Solid Edge part; units mm, degrees
sketch "Sketch1" plane through (0, 0, 0) normal (0, 0, 1) x (1, 0, 0)
  circle A0 centre (0, 0) radius 32
extrude "Protrusion1" add sketch "Sketch1" against normal blind 8
sketch "Sketch2" plane through (0, 0, 0) normal (0, 0, 1) x (1, 0, 0)
  circle A0 centre (0, 0) radius 10
extrude "nucleo" add sketch "Sketch2" along normal blind 3
sketch "Sketch3" plane through (0, 0, -8) normal (0, 0, -1) x (-1, 0, 0)
  line L0 (-9.0257, 1.3213) -> (-30.1049, -10.8488)
  arc A0 (-31.3249, -6.5384) -> (-30.1049, -10.8488) centre (0, 0) ccw
  line L1 (-15, 2.8868) -> (-31.3249, -6.5384)
  arc A1 (-10, 11.547) -> (-15, 2.8868) centre (-20, 11.547) cw
  line L2 (-10, 30.3974) -> (-10, 11.547)
  arc A2 (-5, 31.607) -> (-10, 30.3974) centre (0, 0) ccw
  line L3 (-5, 31.607) -> (-5, 11.547)
  arc A3 (-5, 11.547) -> (-9.0257, 1.3213) centre (-20, 11.547) cw
  line L4 (13.4645, 3.821) -> (31.3338, -6.4958)
  arc A4 (29.8227, -11.6019) -> (31.3338, -6.4958) centre (0, 0) ccw
  line L5 (29.8227, -11.6019) -> (12.5, -1.6006)
  arc A5 (12.5, -1.6006) -> (5, 11.3898) centre (20, 11.3898) cw
  line L6 (5, 11.3898) -> (5, 31.607)
  arc A6 (10, 30.3974) -> (5, 31.607) centre (0, 0) ccw
  line L7 (10, 30.3974) -> (10, 11.3898)
  arc A7 (10, 11.3898) -> (13.4645, 3.821) centre (20, 11.3898) ccw
  line L8 (7.748, -9.9604) -> (25.0296, -19.9379)
  arc A8 (21.3573, -23.8299) -> (25.0296, -19.9379) centre (0, 0) ccw
  line L9 (3.3929, -13.4582) -> (21.3573, -23.8299)
  arc A9 (-4.752, -14.2906) -> (3.3929, -13.4582) centre (0.248, -22.9508) cw
  line L10 (-21.3249, -23.8589) -> (-4.752, -14.2906)
  arc A10 (-24.8724, -20.1336) -> (-21.3249, -23.8589) centre (0, 0) ccw
  line L11 (-24.8724, -20.1336) -> (-7.252, -9.9604)
  arc A11 (-7.252, -9.9604) -> (7.748, -9.9604) centre (0.248, -22.9508) cw
extrude "paredes" add sketch "Sketch3" along normal blind 19
sketch "Sketch4" plane through (0, 0, 0) normal (0, 0, 1) x (1, 0, 0)
  circle A0 centre (0, 0) radius 10
extrude "VaciadoExtruido_3" cut sketch "Sketch4" along normal mid plane 58
hole "Agujero_1" at (6.4705, -24.1481, -8) direction (0, 0, 1) diameter 9.5 depth 4.75
hole "Hole1" [suppressed]
hole "Agujero_3" at (6.4705, -24.1481, -3.25) direction (0, 0, 1) diameter 5.5 end through all
hole "Agujero_6" at (14.3967, -19.8589, -19) direction (0.5, 0.866, 0) diameter 6 end through all
hole "Agujero_7" at (-24.4055, -2.4958, -19) direction (0.5, -0.866, 0) diameter 6 end through all
hole "Agujero_8" at (10, 22.3974, -19) direction (-1, 0, 0) diameter 6 end through all
chamfer "CHAFLAN" distance 2.75 distance2 3 2 edges at (7.5243, 31.1028, -27) (30.7904, -8.715, -27) measured on face at (9.1242, 10.8036, -27)
chamfer "Chaflán_2" distance 2.75 distance2 3 2 edges at (-7.5243, 31.1028, -27) (-30.6846, -9.0804, -27) measured on face at (-18.4302, -3.9683, -27)
chamfer "Chaflán_3" distance 2.75 distance2 3 2 edges at (-23.2749, -21.9608, -27) (23.1736, -22.0677, -27) measured on face at (-17.2116, -21.1809, -27)
pattern_circular "Pattern1" count 3 over 360 about axis through (0, 0, -8) along (0, 0, 1) of "Agujero_1", "Agujero_3"
The model under review builds one solid part; all positions refer to its coordinate system, in mm. A direction names the side the tool comes from. Give positions to 0.01 mm unless a question says otherwise; leave off trailing zeros. Write each loop counter-clockwise with the first axis right and the second up, starting at its lowest first coordinate (ties: lowest second). Pieces come first, ordered by that corner, then holes. Notation, with made-up numbers: (17.5, 46) -> (69.5, 46) arc R16 cw to (69.5, 70) -> close; hole circle Ø8 at (1, -28.5). An arc over 180 degrees is marked (long way). Put each result on its own line as item: value.
(1) The part is to be moulded in two halves that separate along X. For faces 1 (the flat face through (-12, 5, -27)), 2 (the conical face through (21.832, -21.505, -25.479)), 3 (the cylindrical face through (-11.22, -0.77, -17.37)), 4 (the flat face through (-21.28, -6.67, -15.26)), say which applies: pulls with the +X half, pulls with the -X half, needs draft (parallel to the pull), parting line crosses it, or undercut.
Results are:
face 1: needs draft
face 2: pulls with the +X half
face 3: undercut
face 4: undercut
(2) Tool access review of faces 5 (the cylindrical face through (0.83, -13.01, -17.37)), 6 (the flat face through (-10, 21, -15)), 7 (the cylindrical face through (6.041, -9.333, -17.367)), 8 (the flat face through (21.23, -0.71, -17.37)): name each direction out of +Z, -Z, +X, -X, +Y, -Y from which nothing blocks a thin tool from reaching the whole face with its end or side.
Results are:
face 5: -Z, -Y
face 6: -Z, -X, +Y
face 7: -Z
face 8: -Z, +X, +Y
(3) We need section A-A, the plane z = -10. State how many separate pieces and enclosed holes the cut face has, and give its area (3 significant figures).
Results are:
separate pieces: 3
enclosed holes: 0
area: 738 mm²
(4) For pin 1 Ø5 at (y, z) = (-17.5, -3.5) entering from -X; pin 2 Ø21 at (x, y) = (2, -27) entering from -Z; pin 3 Ø6 at (x, z) = (1.5, -22.5) entering from +Y; pin 4 Ø5 at (y, z) = (22.4, -19) entering from -X, all flat-tipped, find the tip position at first contact; note any pin that passes through.
Results are:
pin 1: x = -28.27
pin 2: z = -8
pin 3: y = -8.93
pin 4: through
(5) To check wall thickness, follow probe 1 along X at (y, z) = (26.5, -24.5); probe 2 along Y at (x, z) = (8.6, -19); probe 3 along Z at (x, y) = (-11.5, -10). State the ranges of each line that lie inside material, in increasing order. Write a range as from..to.
Results are:
probe 1: -10..-5, 5..10
probe 2: -16.51..-10.74, 5.1..19.4, 25.4..30.82
probe 3: -8..0
(6) We need section B-B, the plane x = 0. Give the boundary of the cut face in (y, z), and give its area (3 significant figures).
Results are:
outline: (-32, -8) -> (-12.95, -8) -> (-12.95, -27) -> (-10, -27) -> (-10, 0) -> (-32, 0) -> close; (10, -8) -> (32, -8) -> (32, 0) -> (10, 0) -> close
area: 408 mm²
